For this review, use the dimensioned drawing (mm, ordinates from the lowest corner) and the shaded views. A direction names the side the tool comes from. Give positions to 0.01 mm unless a question says otherwise; leave off trailing zeros. Write each loop counter-clockwise with the first axis right and the second up, starting at its lowest first coordinate (ties: lowest second). Pieces come first, ordered by that corner, then holes.
1) For P1, Ø3, axis at x = 25, z = 15, coming from the +Y side; P2, Ø1.5, axis at y = 1.5, z = 22, coming from the -X side; P3, Ø0.9, axis at y = 1.5, z = 7, coming from the +X side, all flat-tipped, find the tip position at first contact; note any pin that passes through.
2) Wall thickness on line 1 along Z through (x, y) = (15, 1.25); line 2 along X through (y, z) = (2.3, 15): over which ranges is each line inside the solid? List them lowest first.
3) We need section A-A on z = 5. Give the boundary of the cut face in (x, y), and give its area (3 significant figures).
4) We need section D-D on x = 25. Give the boundary of the cut face in (y, z), and give its area (3 significant figures).
5) We need section C-C on y = 0.5. Give the boundary of the cut face in (x, z).
6) We need section B-B on x = 15. Give the boundary of the cut face in (y, z).
7) Machinability: for the marked faces 1, 2 and 3, which of the approach directions +Z, -Z, +X, -X, +Y, -Y give a long, thin tool a straight path to every point of the face, cutting with its end or side? Answer none if there is none.
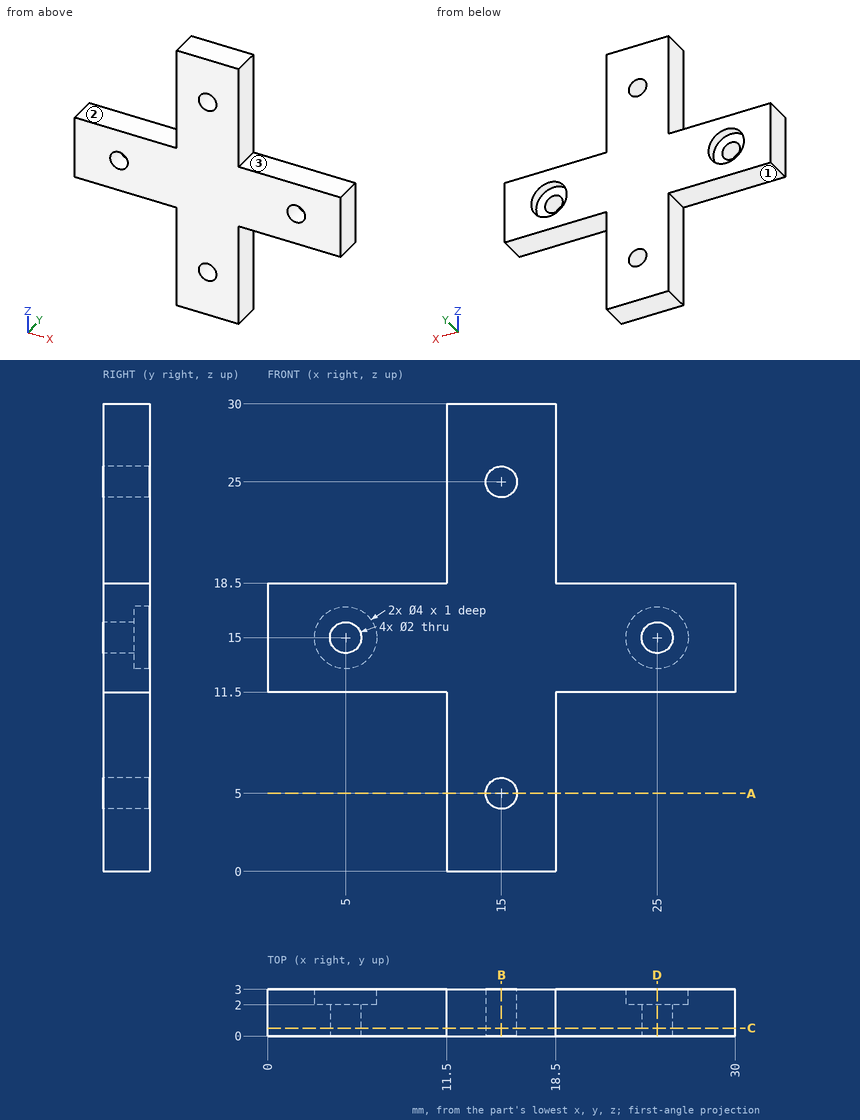
Results list:
1. P1: stops at y = 2
1. P2: stops at x = 11.5
1. P3: stops at x = 18.5
2. line 1: z = 0 to 4, 6 to 24, 26 to 30
2. line 2: x = 0 to 3, 7 to 23, 27 to 30
3. outline: (11.5, 0) - (14, 0) - (14, 3) - (11.5, 3) - close; (16, 0) - (18.5, 0) - (18.5, 3) - (16, 3) - close
3. area: 15.0 mm2
4. outline: (0, 11.5) - (3, 11.5) - (3, 13) - (2, 13) - (2, 14) - (0, 14) - close; (0, 16) - (2, 16) - (2, 17) - (3, 17) - (3, 18.5) - (0, 18.5) - close
4. area: 13.0 mm2
5. outline: (0, 11.5) - (11.5, 11.5) - (11.5, 0) - (18.5, 0) - (18.5, 11.5) - (30, 11.5) - (30, 18.5) - (18.5, 18.5) - (18.5, 30) - (11.5, 30) - (11.5, 18.5) - (0, 18.5) - close; hole circle Ø2 at (5, 15); hole circle Ø2 at (15, 5); hole circle Ø2 at (15, 25); hole circle Ø2 at (25, 15)
6. outline: (0, 0) - (3, 0) - (3, 4) - (0, 4) - close; (0, 6) - (3, 6) - (3, 24) - (0, 24) - close; (0, 26) - (3, 26) - (3, 30) - (0, 30) - close
7. face 1: -Z, -X, +Y, -Y
7. face 2: +Z, -X, +Y, -Y
7. face 3: +Z, +X, +Y, -Y
